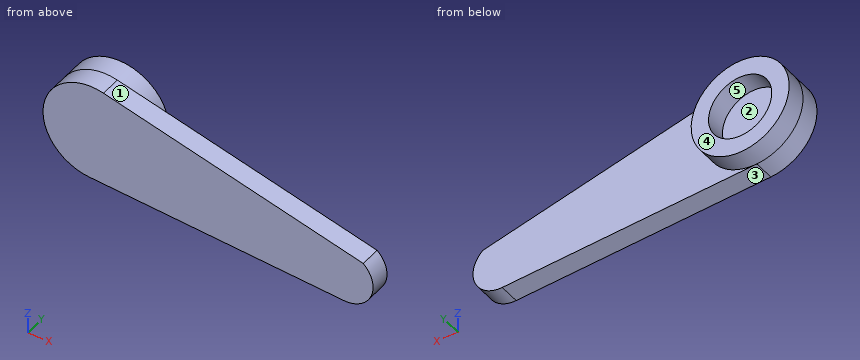
from build123d import *
from build123d.topology import SkipClean

# Parameters (mm, degrees)
BOSS_EXTRUDE1_DEPTH = 1.3
SKETCH2_R           = 3.1
SKETCH2_R_2         = 2
BOSS_EXTRUDE2_DEPTH = 1.3


with BuildPart() as part:
    # Sketch1 → Boss-Extrude1 (new body)
    with BuildSketch(Plane(origin=(0, 0, 0), x_dir=(1, 0, 0), z_dir=(0, 1, 0))):
        with BuildLine():
            Line((-0.178960564, 3.094830063), (15.932363725, 4.026477881))
            ThreePointArc((15.932363725, 4.026477881), (17.659689309, 2.925654907), (17.159069655, 0.939491555))
            Line((17.159069655, 0.939491555), (0.725076499, -3.014011292))
            ThreePointArc((0.725076499, -3.014011292), (-3.066601756, -0.453821189), (-0.178960564, 3.094830063))
        make_face()
    extrude(amount=BOSS_EXTRUDE1_DEPTH)

    # Sketch2 → Boss-Extrude2 (add)
    with SkipClean():  # the faces are left unmerged after this step: merging them gives an invalid solid
        with BuildSketch(Plane(origin=(0, 1.3, 0), x_dir=(1, 0, 0), z_dir=(0, 1, 0))):
            with Locations(Location((0, 0, 0), (0, 0, 93.309480289))):
                Circle(SKETCH2_R)
            with Locations(Location((0, 0, 0), (0, 0, 270))):
                Circle(SKETCH2_R_2, mode=Mode.SUBTRACT)
        extrude(amount=BOSS_EXTRUDE2_DEPTH)


solid = part.part
Could you check a few things on this model? Use its own coordinates, in mm. Face numbers are marked on the shaded views. A direction names the side the tool comes from. Give positions to 0.01 mm unless a question says otherwise; leave off trailing zeros. Order: outer loops, then holes, each group sorted by start corner. A loop starts at its lowest first (then second) coordinate and runs counter-clockwise, first axis right, second up. Notation, with made-up numbers: (14.5, 27) - (49.5, 27) arc R19 ccw to (49.5, 54) - close; hole circle Ø10 at (7.25, -11.75). An arc over 180 degrees is marked (long way). Return JSON: item names as keys, results as strings. Group by question number.
Q1. Suppose I cut it at B-B, the plane z = 0. Please give me the cut outline in (x, y).
Q2. Suppose I cut it at C-C, the plane y = 1. Please give me the cut outline in (x, z).
Q3. Thinking about a two-plate mould opening in X: for the marked faces 3, 4 and 5, which applies, pulls with the +X half, pulls with the -X half, needs draft (parallel to the pull), parting line crosses it, or undercut?
Q4. Please list where these lines run through material, in increasing order: line 1 along X through (y, z) = (1.75, 0); line 2 along Y through (x, z) = (4.5, 1); line 3 along X through (y, z) = (1.35, 1.25). Write a range as [from, to].
Q5. Which directions (+Z, -Z, +X, -X, +Y, -Y) give clear straight access to the entire face, cutting with the end or side of a thin tool? Please do the marked faces 1 and 2.
Q6. Suppose I cut it at D-D, the plane x = 6. Please give me the cut outline in (y, z).
Q7. Will this pin go through, and if not, where does the flat tip stop? pin 1 Ø2 at (x, z) = (6.5, -1.5) entering from +Y.
Resolved:
{
 "1": {"outline": "(-3.1, 0) - (13.25, 0) - (13.25, 1.3) - (3.1, 1.3) - (3.1, 2.6) - (2, 2.6) - (2, 1.3) - (-2, 1.3) - (-2, 2.6) - (-3.1, 2.6) - close"},
 "2": {"outline": "(-0.18, -3.09) - (15.93, -4.03) arc R1.75 ccw to (17.16, -0.94) - (0.73, 3.01) arc R3.1 ccw (long way) to start"},
 "3": {"face 3": "pulls with the -X half", "face 4": "needs draft", "face 5": "undercut"},
 "4": {"line 1": "x = [-3.1, -2], [2, 3.1]", "line 2": "y = [0, 1.3]", "line 3": "x = [-2.84, -1.56], [1.56, 2.84]"},
 "5": {"face 1": "+Z, +X, +Y, -Y", "face 2": "+Y"},
 "6": {"outline": "(0, -3.45) - (1.3, -3.45) - (1.3, 1.75) - (0, 1.75) - close"},
 "7": {"pin 1": "stops at y = 1.3"}
}
